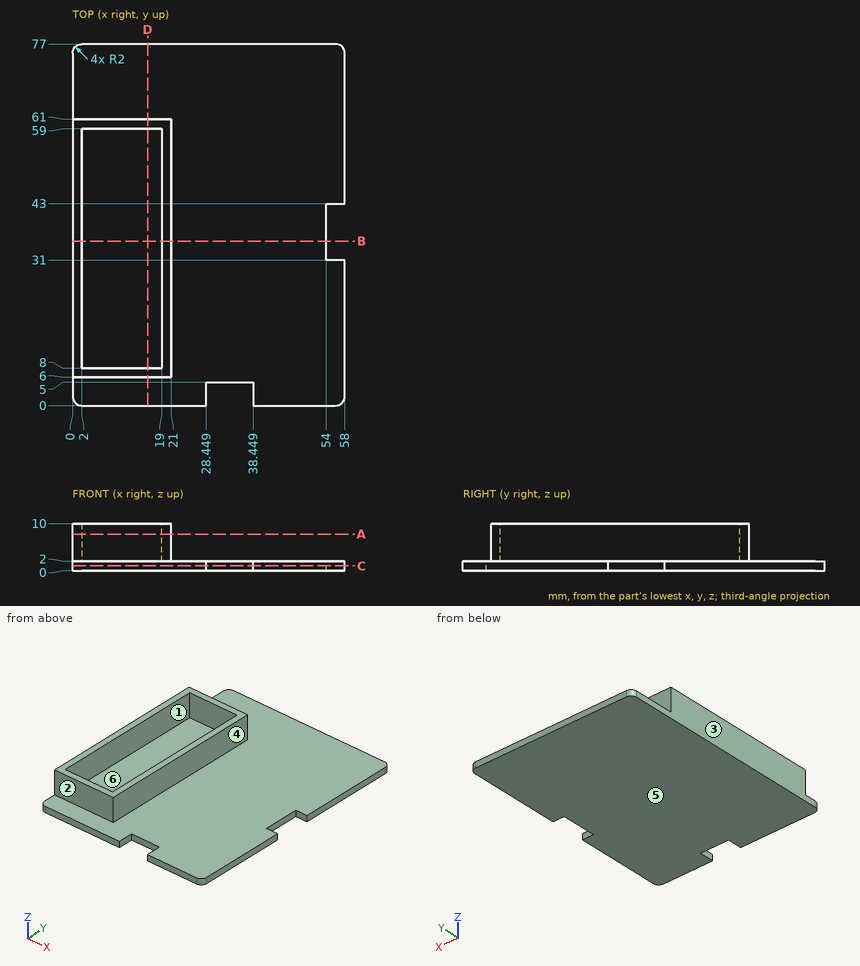
Input: dimensioned drawing with shaded views. Units: mm. Origin: part minimum x, y, z. A direction names the side the tool comes from. Round coordinates to 2 decimals unless told otherwise and drop trailing zeros. Loops run counter-clockwise (first coordinate to the right, second up) from the corner with the lowest first, then second, coordinate; pieces in that order, holes last. Notation, with made-up numbers: (41, 53.5) -> (73, 53.5) arc R18 ccw to (73, 60.5) -> close; hole circle Ø2 at (-8.5, -33). An arc over 180 degrees is marked (long way). One line per item, written item: value.
(1) Pin query (flat end, axial travel): pin 1 (1 mm diameter, centred on y = 62, z = 6.5, fed in from +X); pin 2 (5 mm diameter, centred on x = 14.5, y = 23, fed in from +Z); pin 3 (2 mm diameter, centred on x = 12.5, z = 3.5, fed in from -Y); pin 4 (0.6 mm diameter, centred on y = 1.5, z = 1.5, fed in from -X). Return the tip coordinate at first contact, or that it passes through.
Geometry check:
pin 1: through
pin 2: z = 2
pin 3: y = 6
pin 4: x = 0.01
(2) Section B-B (y = 35). Return the cut outline in (x, z), plus the area to 3 significant figures.
Geometry check:
outline: (0, 0) -> (54, 0) -> (54, 2) -> (21, 2) -> (21, 10) -> (19, 10) -> (19, 2) -> (2, 2) -> (2, 10) -> (0, 10) -> close
area: 140 mm2
(3) Mould query, pull axis Y, two halves, no side actions, for the marked faces 1, 2 and 3. Classes: pulls with the +Y half, pulls with the -Y half, needs draft (parallel to the pull), parting line crosses it, or undercut.
Geometry check:
face 1: undercut
face 2: pulls with the -Y half
face 3: needs draft
(4) Material intervals for line 1 (X direction, y = 57, z = 2.5); line 2 (Y direction, x = 5.5, z = 8.75); line 3 (Y direction, x = 55, z = 1), sorted ascending. Write a range as [from, to].
Geometry check:
line 1: [0, 2], [19, 21]
line 2: [6, 8], [59, 61]
line 3: [0, 31], [43, 77]
(5) Section A-A (z = 7.75). Return the cut outline in (x, y).
Geometry check:
outline: (0, 6) -> (21, 6) -> (21, 61) -> (0, 61) -> close; hole (2, 8) -> (19, 8) -> (19, 59) -> (2, 59) -> close
(6) Section C-C (z = 1). Return the cut outline in (x, y), plus the area to 3 significant figures.
Geometry check:
outline: (0, 2) arc R2 ccw to (2, 0) -> (28.45, 0) -> (28.45, 5) -> (38.45, 5) -> (38.45, 0) -> (56, 0) arc R2 ccw to (58, 2) -> (58, 31) -> (54, 31) -> (54, 43) -> (58, 43) -> (58, 75) arc R2 ccw to (56, 77) -> (2, 77) arc R2 ccw to (0, 75) -> close
area: 4,360 mm2
(7) Set-up query: the marked faces 4, 5 and 6. Return all of +Z, -Z, +X, -X, +Y, -Y with unobstructed straight access to the full face (end or side cutting, diameter ignored); none if empty.
Geometry check:
face 4: +Z, +X, +Y, -Y
face 5: -Z, +X, -X, +Y, -Y
face 6: +Z
(8) Section D-D (x = 16). Return the cut outline in (y, z).
Geometry check:
outline: (0, 0) -> (77, 0) -> (77, 2) -> (61, 2) -> (61, 10) -> (59, 10) -> (59, 2) -> (8, 2) -> (8, 10) -> (6, 10) -> (6, 2) -> (0, 2) -> close
